Can you work these out from the model? Positions are in its coordinate system, mm. A direction names the side the tool comes from. Round coordinates to 2 decimals unless told otherwise and drop trailing zeros. Order: outer loops, then holes, each group sorted by start corner. A loop starts at its lowest first (then second) coordinate and runs counter-clockwise, first axis right, second up. Notation, with made-up numbers: (47.5, 60.25) -> (89.5, 60.25) arc R27 ccw to (89.5, 90.25) -> close; hole circle Ø9 at (9.25, -21). An arc over 180 degrees is marked (long way). Use a Markdown table: item, result. Add a question column.
Q1. I need wall thicknesses on line 1 along Z through (x, y) = (12.7, 0.8); line 2 along Z through (x, y) = (-38, 172.5); line 3 along Z through (x, y) = (12.7, 2.05). Which ranges of each line are inside material? Lowest first, please. Write a range as [from, to].
Q2. If we section it at A-A on y = 137: List the corners of the cut face in (x, z) for me, plus the area to 3 significant figures.
Q3. For faces 5 (the face through (-102.11, 240.9, 68.3)), 6 (the face through (104.146, 250.869, 35.329)), 7 (the face through (10, 3.048, -13)), 8 (the face through (-85, 262, 66.802)), which set-ups out of +Z, -Z, +X, -X, +Y, -Y let a thin tool reach every point of the face, with its end or its side?
Q4. We'd pull the mould along X, two halves only. Please class faces 1 (the face through (102.187, 247.477, 3.965)), 2 (the face through (127.51, 240.9, 68.35)), 3 (the face through (26.2, 128, 0)), 4 (the face through (-79.2, 251.66, 65.93)): +X half, -X half, draft (parallel to the pull), parting line (faces both ways), or undercut.
Q5. If we section it at B-B on y = 50: List the corners of the cut face in (x, z) for me, plus the area to 3 significant figures.
Q6. I'm going to push flat-ended pins straight in: pin 1 Ø12 at (x, y) = (-49, 197) entering from +Z; pin 2 Ø5 at (y, z) = (249, 21.5) entering from +X; pin 3 Ø9.5 at (x, z) = (17, -16.5) entering from +Y. Where does each tip first touch, or does it pass through?
Q7. If we section it at C-C on x = 46.5: List the corners of the cut face in (y, z) for me, plus the area to 3 significant figures.
Autodesk Inventor part; units mm, degrees
ref_plane "YZ Plane" through (0, 0, 0) normal (1, 0, 0) x (0, 1, 0)
ref_plane "XZ Plane" through (0, 0, 0) normal (0, 1, 0) x (-1, 0, 0)
ref_plane "XY Plane" through (0, 0, 0) normal (0, 0, 1) x (1, 0, 0)
sketch "Sketch13" plane through (0, 0, 0) normal (0, 0, 1) x (1, 0, 0)
  line L0 (0, 0) -> (25.4, 0)
  line L1 (25.4, 0) -> (25.4, 101.6)
  line L2 (0, 0) -> (0, 101.6)
  line L3 (0, 101.6) -> (-84.322, 247.65)
  line L4 (25.4, 101.6) -> (166.7245, 101.6) construction
  line L5 (25.4, 101.6) -> (109.722, 247.65)
  line L6 (25.4, 101.6) -> (194.044, 101.6) construction
  line L7 (-84.322, 247.65) -> (-73.3235, 254)
  line L8 (109.722, 247.65) -> (98.7235, 254)
  line L9 (-73.3235, 254) -> (12.7, 105.003)
  line L10 (98.7235, 254) -> (12.7, 105.003)
  dimension "d54" = 25.4
  dimension "d55" = 101.6
  dimension "d133" = 60
  dimension "d134" = 150
  dimension "d135" = 12.7
  dimension "d137" = 12.7
  dimension "d139" = 0
  dimension "d140" = 152.4
  dimension "d141" = 152.4
extrude "Plate5" add sketch "Sketch13" along normal blind 3.048
ref_plane "Work Plane1" through (0, 0, 25.4) normal (0, -1, 0) x (1, 0, 0)
sketch "Sketch20" plane through (0, 3.048, 3.048) normal (0, -1, 0) x (1, 0, 0)
  line L0 (25.4, 0) -> (0, 0)
  line L1 (0, 0) -> (0, -25.4)
  line L2 (0, -25.4) -> (25.4, -25.4)
  line L3 (25.4, -25.4) -> (25.4, 0)
edge flange "Flange7" height 25.4 angle 90 thickness 3.048 bend radius 3.048 thickness toward (0, -1, 0) relief tear relief width 3.048 relief depth 1.524 edges at (12.7, 0, 0) wall of the first edge with corners at (25.4, 3.048, 3.048) (0, 3.048, 3.048) (0, 3.048, -22.352) (25.4, 3.048, -22.352)
bend "Bend7"
corner "Corner7"
sketch "Sketch21" plane through (0, 0, -22.352) normal (0, -1, 0) x (1, 0, 0)
  line L0 (25.4, 0) -> (0, 0)
  line L1 (25.4, 19.304) -> (25.4, 0)
  circle A0 centre (12.7, 9.652) radius 2.54
  point P0 (0, 22.352)
  dimension "d123" = 5.08
  dimension "d124" = 12.7
  dimension "d125" = 9.652
extrude "Cut3" cut sketch "Sketch21" against normal blind 3.048
sketch "Sketch24" plane through (-82.798, 245.0104, 0) normal (-0.5, 0.8660254, 0) x (-0.8660254, -0.5, 0)
  line L0 (-12.7, 0) -> (0, 0)
  line L1 (0, 0) -> (0, 69.85)
  line L2 (0, 69.85) -> (-12.7, 69.85)
  line L3 (-12.7, 69.85) -> (-12.7, 0)
edge flange "Flange8" height 69.85 angle 90 thickness 3.048 bend radius 3.048 thickness toward (-0.5, 0.8660254, 0) relief tear relief width 3.048 relief depth 1.524 corner gap 3.048 corner form 0 edges at (-78.8227, 250.825, 3.048) (104.2227, 250.825, 3.048) wall of the first edge with corners at (-71.7995, 251.3604, 0) (-82.798, 245.0104, 0) (-82.798, 245.0104, 69.85) (-71.7995, 251.3604, 69.85)
bend "Bend8"
corner "Corner8"
sketch "Sketch25" plane through (-71.7995, 251.3604, 66.802) normal (0, 0, 1) x (1, 0, 0)
  line L0 (-10.9985, -6.35) -> (0, 0)
  line L1 (0, 0) -> (-12.7, 21.997)
  line L2 (-12.7, 21.997) -> (-23.6985, 15.647)
  line L3 (-23.6985, 15.647) -> (-10.9985, -6.35)
edge flange "Flange9" height 25.4 angle 90 thickness 3.048 bend radius 3.048 thickness toward (0, 0, 1) relief tear relief width 3.048 relief depth 1.524 corner gap 3.048 corner form 0 edges at (-78.8227, 250.825, 69.85) (104.2227, 250.825, 69.85) wall of the first edge with corners at (-82.798, 245.0104, 66.802) (-71.7995, 251.3604, 66.802) (-84.4995, 273.3574, 66.802) (-95.498, 267.0074, 66.802)
bend "Bend9"
corner "Corner9"
sketch "Sketch26" plane through (-84.4995, 273.3574, 69.85) normal (0.8660254, 0.5, 0) x (0, 0, -1)
  line L0 (0, -19.304) -> (3.048, -19.304)
  line L1 (3.048, 0) -> (3.048, -19.304)
  line L2 (3.048, 0) -> (0, 0)
  line L3 (0, 0) -> (0, -19.304)
  point P0 (69.85, -278.9842)
extrude "Extrusion10" add sketch "Sketch26" along normal blind 38.1
sketch "Sketch27" plane through (120.898, 267.0074, 69.85) normal (0.8660254, -0.5, 0) x (0, 0, -1)
  line L0 (0, -19.304) -> (3.048, -19.304)
  line L1 (3.048, 0) -> (3.048, -19.304)
  line L2 (3.048, 0) -> (0, 0)
  line L3 (0, 0) -> (0, -19.304)
  point P0 (69.85, -291.6842)
extrude "Extrusion11" add sketch "Sketch27" along normal blind 38.1
sketch "Sketch28" plane through (-95.498, 267.0074, 66.802) normal (-0.8660254, -0.5, 0) x (0, 0, 1)
  line L0 (0, -19.304) -> (3.048, -19.304)
  line L1 (3.048, -19.304) -> (3.048, 0)
  line L2 (0, 0) -> (3.048, 0)
  line L3 (0, 0) -> (0, -19.304)
  point P0 (-66.802, -278.9842)
extrude "Extrusion12" add sketch "Sketch28" along normal blind 38.1
sketch "Sketch29" plane through (109.8995, 273.3574, 66.802) normal (-0.8660254, 0.5, 0) x (0, 0, 1)
  line L0 (0, -19.304) -> (3.048, -19.304)
  line L1 (3.048, -19.304) -> (3.048, 0)
  line L2 (0, 0) -> (3.048, 0)
  line L3 (0, 0) -> (0, -19.304)
  point P0 (-66.802, -291.6842)
extrude "Extrusion13" add sketch "Sketch29" along normal blind 38.1
equation "\"d126\" = Thickness"
equation "\"d113\" = BendReliefWidth"
equation "\"d114\" = BendReliefDepth"
equation "\"d115\" = MinimumRemnant"
equation "\"d116\" = BendRadius"
equation "\"d119\" = BendRadius"
equation "\"d120\" = CornerReliefSize"
equation "\"d121\" = GapSize"
equation "\"d122\" = JacobiRadiusSize"
equation "\"d142\" = BendReliefWidth"
equation "\"d143\" = BendReliefDepth"
equation "\"d144\" = MinimumRemnant"
equation "\"d145\" = BendRadius"
equation "\"d148\" = BendRadius"
equation "\"d149\" = CornerReliefSize"
equation "\"d150\" = GapSize"
equation "\"d151\" = JacobiRadiusSize"
equation "\"d152\" = BendReliefWidth"
equation "\"d153\" = BendReliefDepth"
equation "\"d154\" = MinimumRemnant"
equation "\"d155\" = BendRadius"
equation "\"d158\" = BendRadius"
equation "\"d159\" = CornerReliefSize"
equation "\"d160\" = GapSize"
equation "\"d161\" = JacobiRadiusSize"
equation "\"BendRadius\" = Thickness"
equation "\"BendReliefWidth\" = Thickness"
equation "\"BendReliefDepth\" = 0.5 * Thickness"
equation "\"CornerReliefSize\" = 4 * Thickness"
equation "\"MinimumRemnant\" = 2 * Thickness"
equation "\"TransitionRadius\" = BendRadius"
equation "\"JacobiRadiusSize\" = BendRadius"
equation "\"GapSize\" = Thickness"
equation "\"d2\" = BendRadius"
equation "\"d69\" = BendRadius"
properties part number "Feeder-Grabber_v2" material "Aluminum 6061"
Answer below:
| question | item | result |
|---|---|---|
| 1 | line 1 | [-22.35, -15.24], [-10.16, -0.03] |
| 1 | line 2 | [0, 3.05] |
| 1 | line 3 | [-22.35, -15.24], [-10.16, 1.51] |
| 2 | outline | (-20.44, 0) -> (-5.77, 0) -> (-5.77, 3.05) -> (-20.44, 3.05) -> close; (31.17, 0) -> (45.84, 0) -> (45.84, 3.05) -> (31.17, 3.05) -> close |
| 2 | area | 89.4 mm² |
| 3 | face 5 | +Z, -Z, -Y |
| 3 | face 6 | -Z, +X, +Y |
| 3 | face 7 | -Z, +X, -X, +Y |
| 3 | face 8 | -Z, -X, +Y |
| 4 | face 1 | undercut |
| 4 | face 2 | undercut |
| 4 | face 3 | draft |
| 4 | face 4 | -X half |
| 5 | outline | (0, 0) -> (25.4, 0) -> (25.4, 3.05) -> (0, 3.05) -> close |
| 5 | area | 77.4 mm² |
| 6 | pin 1 | z = 3.05 |
| 6 | pin 2 | x = 109.72 |
| 6 | pin 3 | y = 3.05 |
| 7 | outline | (138.15, 0) -> (163.55, 0) -> (163.55, 3.05) -> (138.15, 3.05) -> close |
| 7 | area | 77.4 mm² |
